Here's the drawing with two shaded views (mm, measured from the low corner). I have some questions. Round coordinates to 2 decimals unless told otherwise and drop trailing zeros. Order: outer loops, then holes, each group sorted by start corner. A loop starts at its lowest first (then second) coordinate and runs counter-clockwise, first axis right, second up. Notation, with made-up numbers: (10.5, -13.75) -> (49.5, -13.75) arc R29 ccw to (49.5, 10.25) -> close; hole circle Ø2 at (-14.75, -27.5). An arc over 180 degrees is marked (long way). Answer in a Markdown table with one row per item.
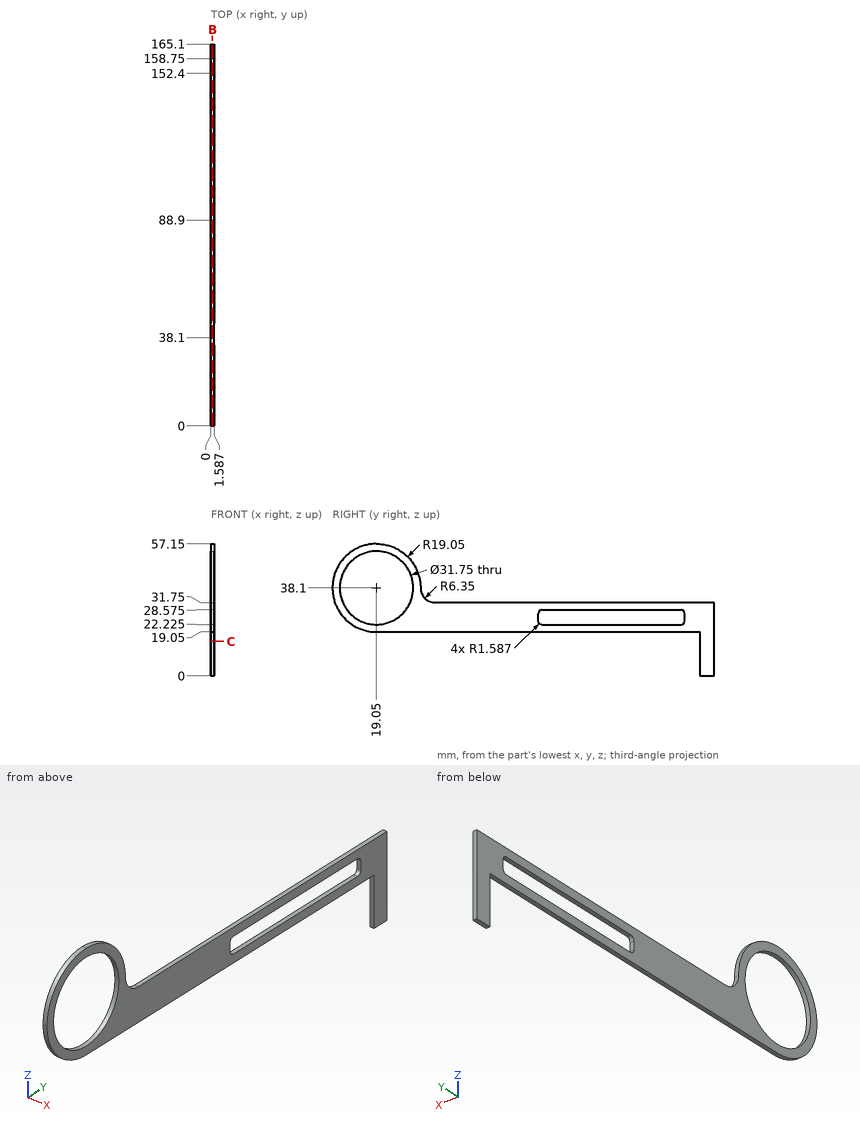
1. For pin 1 Ø6 at (y, z) = (27.5, 44.5) entering from -X (3 decimals); pin 2 Ø0.8 at (x, z) = (1, 26) entering from -Y (1 decimal); pin 3 Ø0.8 at (x, y) = (1, 121.5) entering from +Z; pin 4 Ø0.5 at (x, y) = (1, 134.5) entering from -Z, each with a flat end and sliding along its axis, tell me the tip position at first contact or that it passes through.
Numbers:
| item | result |
|---|---|
| pin 1 | passes through |
| pin 2 | stops at y = 4 |
| pin 3 | stops at z = 31.75 |
| pin 4 | stops at z = 19.05 |
2. Please list where these lines run through material, in increasing order: line 1 along Y through (x, z) = (1.1, 25) (1 decimal); line 2 along Y through (x, z) = (1, 25.5) (1 decimal); line 3 along Y through (x, z) = (0.5, 44) (1 decimal).
Numbers:
| item | result |
|---|---|
| line 1 | y = 5.2 to 10.1, 28 to 88.9, 152.4 to 165.1 |
| line 2 | y = 4.8 to 9.4, 28.7 to 88.9, 152.4 to 165.1 |
| line 3 | y = 0.9 to 4.3, 33.8 to 37.2 |
3. Suppose I cut it at B-B on x = 0.7. State how many separate pieces and enclosed holes the cut face has, then the cut area to 3 significant figures.
Numbers:
| item | result |
|---|---|
| separate pieces | 1 |
| enclosed holes | 2 |
| area | 1,770 mm2 |
4. Suppose I cut it at C-C on z = 15. Write out the boundary of the cut face in (x, y).
Numbers:
| item | result |
|---|---|
| outline | (0, 158.75) -> (1.59, 158.75) -> (1.59, 165.1) -> (0, 165.1) -> close |
